from build123d import *

# Parameters (mm, degrees)
F1_DEPTH = 150
F2_R     = 1.5
F3_DEPTH = 20.001
F4_R     = 1.5
F5_DEPTH = 20.001


with BuildPart() as f1:
    # F0 (on Top) → F1 (new body, symmetric)
    with BuildSketch(Plane.XY):
        Polygon((-20, 0), (0, 0), (0, 20), (-2, 20), (-2, 2), (-20, 2), align=None)
    extrude(amount=F1_DEPTH, both=True)

    # F2 (on face) → F3 (cut, through all)
    with BuildSketch(Plane.YZ):
        with Locations((11, 140)):
            Circle(F2_R)
        with Locations((11, -140)):
            Circle(F2_R)
    extrude(amount=-F3_DEPTH, mode=Mode.SUBTRACT)

    # F4 (on face) → F5 (cut, through all)
    with BuildSketch(Plane.XZ):
        with Locations((-11, 140)):
            Circle(F4_R)
        with Locations((-11, -140)):
            Circle(F4_R)
    extrude(amount=-F5_DEPTH, mode=Mode.SUBTRACT)


solid = f1.part
Source: CAD feature listing. Evaluate the final solid. Frame: model axes, mm. A direction names the side the tool comes from. Give positions to 0.01 mm unless a question says otherwise; leave off trailing zeros. Write each loop counter-clockwise with the first axis right and the second up, starting at its lowest first coordinate (ties: lowest second). Pieces come first, ordered by that corner, then holes. Notation, with made-up numbers: M 20.25,-7 L 53.25,-7 A27 ccw 53.25,13 Z; hole C -13.5,-32.75 d6. An arc over 180 degrees is marked long. Return JSON: item names as keys, results as strings. Group by question number.
1) Cut plane C-C, the plane y = 16. Output: boundary loops of the cut face in (x, z).
2) Ray query, L1, parallel to Z at x = -11, y = 1; L2, parallel to Y at x = -1.15, z = -140; L3, parallel to X at y = 4.25, z = 67.5. Return the intervals inside material, ascending.
3) Set-up query: faces 1 (the face through (-10, 0, 2)), 2 (the face through (-11, 2, 2)). Return all of +Z, -Z, +X, -X, +Y, -Y with unobstructed straight access to the full face (end or side cutting, diameter ignored); none if empty.
4) First-contact query: pin 1 Ø3.5 at (x, z) = (-11, 140) entering from +Y; pin 2 Ø2 at (y, z) = (4, -31.5) entering from -X. Flat tips, straight axial feed; report the tip coordinate or a pass-through.
5) Cut plane A-A, the plane x = -15. Output: boundary loops of the cut face in (y, z), then the cut area to 3 significant figures.
6) Cut plane B-B, the plane z = 112.5. Output: boundary loops of the cut face in (x, y).
Data:
{
 "1": {"outline": "M -2,-150 L 0,-150 L 0,150 L -2,150 Z"},
 "2": {"L1": "z = -150 to -141.5, -138.5 to 138.5, 141.5 to 150", "L2": "y = 0 to 9.5, 12.5 to 20", "L3": "x = -2 to 0"},
 "3": {"face 1": "+Z, -Z, +X, -X, -Y", "face 2": "+Z, -Z, -X, +Y"},
 "4": {"pin 1": "stops at y = 2", "pin 2": "stops at x = -2"},
 "5": {"outline": "M 0,-150 L 2,-150 L 2,150 L 0,150 Z", "area": "600 mm²"},
 "6": {"outline": "M -20,0 L 0,0 L 0,20 L -2,20 L -2,2 L -20,2 Z"}
}
